Check sheet for the drawn part. Datum: minimum x, y, z corner. Units: mm. Round coordinates to 2 decimals unless told otherwise and drop trailing zeros. Write each loop counter-clockwise with the first axis right and the second up, starting at its lowest first coordinate (ties: lowest second). Pieces come first, ordered by that corner, then holes.
Item 1: Cross-section at A-A on x = 1.6. Enter the section's corners in (y, z), plus the area to 3 significant figures.
Item 2: Material ranges on line 1 (Z direction, x = 1.25, y = 65); line 2 (Y direction, x = 2.25, z = 44); line 3 (Y direction, x = 1.65, z = 43.5), recorded low to high.
Item 3: Cross-section at B-B on z = 44. Enter the section's corners in (x, y).
Item 4: Cross-section at D-D on y = 6. Enter the section's corners in (x, z), plus the area to 3 significant figures.
Item 5: Go/stop test with a flat-tipped pin: pin 1 Ø3 at (y, z) = (94, 25) entering from -X. Record where the tip stops, or that it passes through.
Item 6: Cross-section at C-C on y = 65. Enter the section's corners in (x, z).
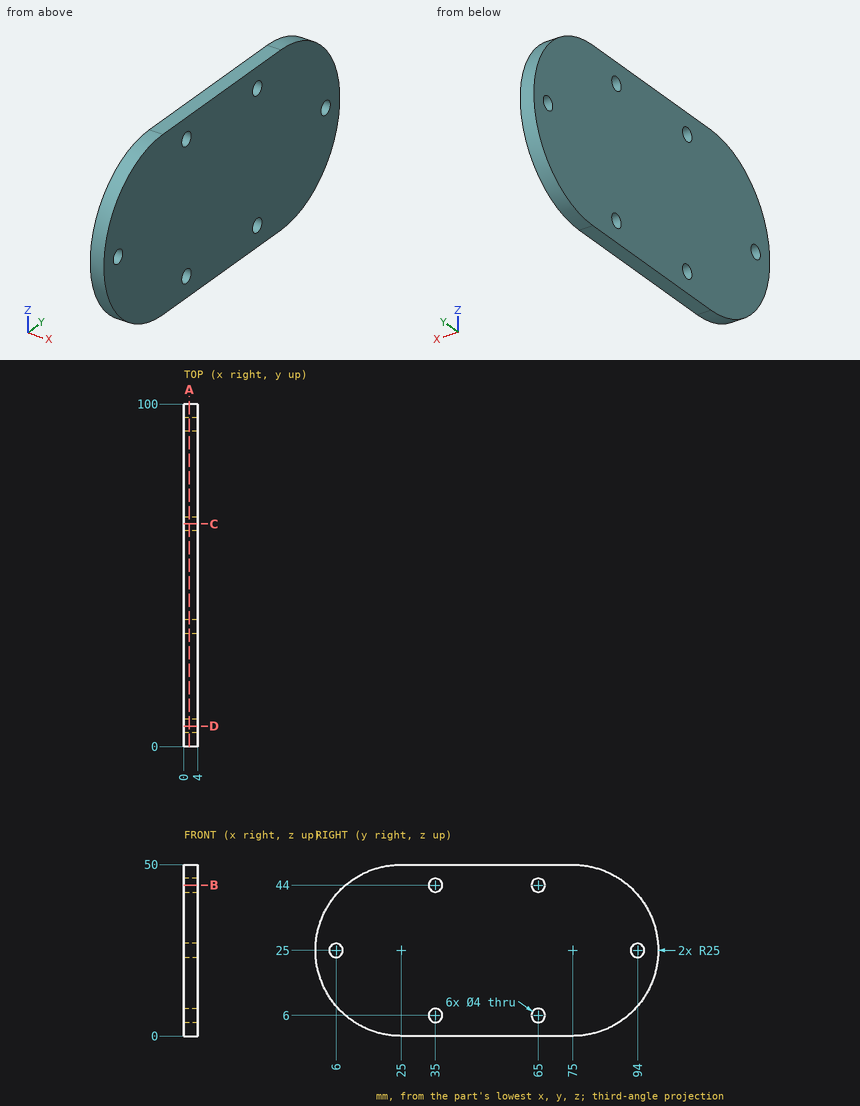
Response values:
1. outline: (25, 0) - (75, 0) arc R25 ccw to (75, 50) - (25, 50) arc R25 ccw to start; hole circle Ø4 at (6, 25); hole circle Ø4 at (35, 6); hole circle Ø4 at (35, 44); hole circle Ø4 at (65, 6); hole circle Ø4 at (65, 44); hole circle Ø4 at (94, 25)
1. area: 4,390 mm2
2. line 1: z = 0 to 4, 8 to 42, 46 to 50
2. line 2: y = 8.75 to 33, 37 to 63, 67 to 91.25
2. line 3: y = 8.18 to 33.06, 36.94 to 63.06, 66.94 to 91.82
3. outline: (0, 8.75) - (4, 8.75) - (4, 33) - (0, 33) - close; (0, 37) - (4, 37) - (4, 63) - (0, 63) - close; (0, 67) - (4, 67) - (4, 91.25) - (0, 91.25) - close
4. outline: (0, 8.75) - (4, 8.75) - (4, 23) - (0, 23) - close; (0, 27) - (4, 27) - (4, 41.25) - (0, 41.25) - close
4. area: 114 mm2
5. pin 1: passes through
6. outline: (0, 0) - (4, 0) - (4, 4) - (0, 4) - close; (0, 8) - (4, 8) - (4, 42) - (0, 42) - close; (0, 46) - (4, 46) - (4, 50) - (0, 50) - close
